Autodesk Inventor part; units mm, degrees
ref_plane "YZ Plane" through (0, 0, 0) normal (1, 0, 0) x (0, 1, 0)
ref_plane "XZ Plane" through (0, 0, 0) normal (0, 1, 0) x (-1, 0, 0)
ref_plane "XY Plane" through (0, 0, 0) normal (0, 0, 1) x (1, 0, 0)
sketch "T-Slot 4040 Base" plane through (0, 0, 0) normal (0, 0, 1) x (1, 0, 0)
  line L0 (-28, 0) -> (28, 0) construction
  line L1 (0, -28) -> (0, 28) construction
  circle A0 centre (0, 0) radius 5.1
  line L2 (-7.5, -7.5) -> (7.5, -7.5)
  line L3 (7.5, -7.5) -> (7.5, 7.5)
  line L4 (7.5, 7.5) -> (-7.5, 7.5)
  line L5 (-7.5, 7.5) -> (-7.5, -7.5)
  line L6 (-7.5, -7.5) -> (7.5, 7.5) construction
  line L7 (7.5, -7.5) -> (-7.5, 7.5) construction
  line L8 (-20, 20) -> (20, 20)
  line L9 (20, 20) -> (20, -20)
  line L10 (20, -20) -> (-20, -20)
  line L11 (-20, -20) -> (-20, 20)
  line L12 (-20, 20) -> (20, -20) construction
  line L13 (20, 20) -> (-20, -20) construction
  line L14 (20, 5) -> (14.5, 5)
  line L15 (14.5, 5) -> (14.5, 10)
  line L16 (14.5, 10) -> (12.4749, 10)
  line L17 (12.4749, 10) -> (7.5, 5.0251)
  line L18 (5, 20) -> (5, 14.5)
  line L19 (5, 14.5) -> (10, 14.5)
  line L20 (10, 14.5) -> (10, 12.4749)
  line L21 (10, 12.4749) -> (5.0251, 7.5)
  line L22 (18.5, 18.5) -> (11.5, 18.5)
  line L23 (11.5, 18.5) -> (11.5, 11.5)
  line L24 (11.5, 11.5) -> (18.5, 11.5)
  line L25 (18.5, 11.5) -> (18.5, 18.5)
  line L26 (18.5, 18.5) -> (11.5, 11.5) construction
  line L27 (11.5, 18.5) -> (18.5, 11.5) construction
  line L28 (3.0732, 1.3088) -> (4.38, 2.6125) construction
  line L29 (5.905, 4.1338) -> (4.1393, 5.9037)
  line L30 (4.1393, 5.9037) -> (2.6122, 4.3802)
  line L31 (1.3075, 3.0787) -> (3.0732, 1.3088) construction
  line L32 (3.0732, 1.3088) -> (4.1393, 5.9037) construction
  line L33 (5.905, 4.1338) -> (1.3075, 3.0787) construction
  line L34 (4.38, 2.6125) -> (5.905, 4.1338)
  line L35 (2.6122, 4.3802) -> (1.3075, 3.0787) construction
  line L36 (-20, 5) -> (-14.5, 5)
  line L37 (-14.5, 5) -> (-14.5, 10)
  line L38 (-14.5, 10) -> (-12.4749, 10)
  line L39 (-12.4749, 10) -> (-7.5, 5.0251)
  line L40 (-5, 20) -> (-5, 14.5)
  line L41 (-5, 14.5) -> (-10, 14.5)
  line L42 (-10, 14.5) -> (-10, 12.4749)
  line L43 (-10, 12.4749) -> (-5.0251, 7.5)
  line L44 (-18.5, 18.5) -> (-11.5, 18.5)
  line L45 (-11.5, 18.5) -> (-11.5, 11.5)
  line L46 (-11.5, 11.5) -> (-18.5, 11.5)
  line L47 (-18.5, 11.5) -> (-18.5, 18.5)
  line L48 (-5.905, 4.1338) -> (-4.1393, 5.9037)
  line L49 (-4.1393, 5.9037) -> (-2.6122, 4.3802)
  line L50 (-4.38, 2.6125) -> (-5.905, 4.1338)
  line L51 (7.5, -7.5) -> (-7.5, -7.5)
  line L52 (20, -5) -> (14.5, -5)
  line L53 (14.5, -5) -> (14.5, -10)
  line L54 (14.5, -10) -> (12.4749, -10)
  line L55 (12.4749, -10) -> (7.5, -5.0251)
  line L56 (5, -20) -> (5, -14.5)
  line L57 (5, -14.5) -> (10, -14.5)
  line L58 (10, -14.5) -> (10, -12.4749)
  line L59 (10, -12.4749) -> (5.0251, -7.5)
  line L60 (18.5, -18.5) -> (11.5, -18.5)
  line L61 (11.5, -18.5) -> (11.5, -11.5)
  line L62 (11.5, -11.5) -> (18.5, -11.5)
  line L63 (18.5, -11.5) -> (18.5, -18.5)
  line L64 (18.5, -18.5) -> (11.5, -11.5) construction
  line L65 (11.5, -18.5) -> (18.5, -11.5) construction
  line L66 (3.0732, -1.3088) -> (4.38, -2.6125) construction
  line L67 (5.905, -4.1338) -> (4.1393, -5.9037)
  line L68 (4.1393, -5.9037) -> (2.6122, -4.3802)
  line L69 (1.3075, -3.0787) -> (3.0732, -1.3088) construction
  line L70 (3.0732, -1.3088) -> (4.1393, -5.9037) construction
  line L71 (5.905, -4.1338) -> (1.3075, -3.0787) construction
  line L72 (4.38, -2.6125) -> (5.905, -4.1338)
  line L73 (2.6122, -4.3802) -> (1.3075, -3.0787) construction
  line L74 (-4.38, -2.6125) -> (-5.905, -4.1338)
  line L75 (-4.1393, -5.9037) -> (-2.6122, -4.3802)
  line L76 (-5.905, -4.1338) -> (-4.1393, -5.9037)
  line L77 (-12.4749, -10) -> (-7.5, -5.0251)
  line L78 (-10, -12.4749) -> (-5.0251, -7.5)
  line L79 (-10, -14.5) -> (-10, -12.4749)
  line L80 (-5, -14.5) -> (-10, -14.5)
  line L81 (-5, -20) -> (-5, -14.5)
  line L82 (-18.5, -18.5) -> (-11.5, -18.5)
  line L83 (-11.5, -18.5) -> (-11.5, -11.5)
  line L84 (-11.5, -11.5) -> (-18.5, -11.5)
  line L85 (-18.5, -11.5) -> (-18.5, -18.5)
  line L86 (-14.5, -10) -> (-12.4749, -10)
  line L87 (-14.5, -5) -> (-14.5, -10)
  line L88 (-20, -5) -> (-14.5, -5)
  point P0 (15, 15)
  point P1 (3.6062, 3.6062)
  point P2 (3.6062, 3.6062)
  point P3 (15, -15)
  point P4 (3.6062, -3.6062)
  point P5 (3.6062, -3.6062)
  dimension "d9" = 10.2
  dimension "d12" = 40
  dimension "d13" = 40
  dimension "d14" = 5.5
  dimension "d15" = 15
  dimension "d16" = 7
  dimension "d17" = 10
  dimension "d20" = 1.75
  dimension "d21" = 7
  dimension "d22" = 2
  dimension "d29" = 1.5
  dimension "d30" = 2.5
extrude "Extrusion1" add sketch "T-Slot 4040 Base" along normal blind 1127 contours L5 L4 L3 L2 | L2 L78 L79 L80 L81 L10 L11 L88 L87 L86 L77 L5 | L2 L3 L55 L54 L53 L52 L9 L10 L56 L57 L58 L59 | L39 L38 L37 L36 L11 L8 L40 L41 L42 L43 L4 L5 | L3 L4 L21 L20 L19 L18 L8 L9 L14 L15 L16 L17
fillet "Rundung1" radius 1 16 edges at (11.5, 18.5, 563.5) (18.5, 18.5, 563.5) (18.5, 11.5, 563.5) (11.5, 11.5, 563.5) (-11.5, 18.5, 563.5) (-18.5, 18.5, 563.5) (-18.5, 11.5, 563.5) (-11.5, 11.5, 563.5) (-18.5, -11.5, 563.5) (-11.5, -11.5, 563.5) (-11.5, -18.5, 563.5) (-18.5, -18.5, 563.5) (11.5, -18.5, 563.5) (11.5, -11.5, 563.5) (18.5, -11.5, 563.5) (18.5, -18.5, 563.5)
fillet "Rundung2" radius 3 4 edges at (20, 20, 563.5) (20, -20, 563.5) (-20, -20, 563.5) (-20, 20, 563.5)
properties part number "T-SLOT 4040 B-Type 1127mm"
Geometry check sheet. Reference: the model listing, model coordinates, mm. Round coordinates to 2 decimals unless told otherwise and drop trailing zeros. One line per question, with ' | ' between items. Start each with the question number.
1. Scan lines: line 1 (X direction, y = -16, z = 845); line 2 (Y direction, x = -14, z = 324.5). Record each from-to range of solid material in increasing order. Write a range as [from, to].
2. Cross-section at A-A on z = 313.5. State how many separate pieces and enclosed holes the cut face has, then the cut area to 3 significant figures.
3. Depth check by flat-ended pin: pin 1 (2 mm diameter, centred on x = -2, z = 871, fed in from -Y). Enter the tip coordinate at first touch or a pass-through.
Taken from the geometry:
1) line 1: [-20, -18.5], [-11.5, -5], [5, 11.5], [18.5, 20] | line 2: [-20, -18.5], [-11.5, -10], [10, 11.5], [18.5, 20]
2) separate pieces: 1 | enclosed holes: 5 | area: 616 mm²
3) pin 1: y = -7.5
